For this review, take the finished solid that the model builds, in its own axes (mm). A direction names the side the tool comes from. Give positions to 0.01 mm unless a question says otherwise; leave off trailing zeros. Order: outer loops, then holes, each group sorted by start corner. A loop starts at its lowest first (then second) coordinate and runs counter-clockwise, first axis right, second up. Notation, with made-up numbers: (81.5, -5) -> (130.5, -5) arc R16 ccw to (130.5, 22) -> close; hole circle Ø3 at (46.25, 34.25). An arc over 180 degrees is marked (long way). Return JSON: item names as keys, results as strings. Group by question number.
1) Add section A-A (x = 58.5). Give the boundary of the cut face in (y, z).
2) Insertion check: P1, Ø10, axis at x = 25, y = 1.5, coming from the -Z side; P2, Ø2.5, axis at x = 59.5, z = -1, coming from the +Y side; P3, Ø1.5, axis at x = 40, z = -7, coming from the -Y side; P4, Ø4, axis at x = 51.5, z = 7.5, coming from the +Y side. Each pin has a flat end and moves straight along its axis. Give the tip position at first contact, or say it passes through.
3) Add section B-B (x = 29.5). Give the boundary of the cut face in (y, z) (1 decimal).
4) To check wall thickness, follow line 1 along X through (y, z) = (5, 3.25); line 2 along Y through (x, z) = (40, 0); line 3 along X through (y, z) = (-7.5, -1.5). State the ranges of each line that lie inside material, in increasing order.
5) The part is to be moulded in two halves that separate along Z. For faces 1 (the face through (55.959, 0, 5)), 2 (the face through (39.7, 6.92, -2.41)), 3 (the face through (55.76, 4.65, -1.03)), say which applies: released by +Z, released by -Z, zero draft, split by the parting line, or undercut.
6) For faces 4 (the face through (58.307, 3.219, -5.474)), 5 (the face through (58.307, -3.131, -5.525)), 6 (the face through (5.398, 0, 0)), 7 (the face through (53.578, -2, 10)), 8 (the face through (0, 4, 4)), list the 3-axis set-ups (+Z, -Z, +X, -X, +Y, -Y) from which the entire face can be reached by the end or side of a thin tool; tool diameter is ignored.
from build123d import *

# Parameters (mm, degrees)
CUT_EXTRUDE1_START = -5.0165
SKETCH2_R          = 8.745419401
CUT_EXTRUDE1_DEPTH = 5.0165
SKETCH3_R          = 2.413
CUT_EXTRUDE2_DEPTH = 11.557
SKETCH4_R          = 3.556
CUT_EXTRUDE3_DEPTH = 62.865


with BuildPart() as part:
    # Sketch1 → Revolve1 (revolve)
    with BuildSketch(Plane.XY, mode=Mode.PRIVATE) as revolve1_sk:
        Polygon((2.24506403, 11.1125), (0, 8.86743597), (0, 4.7625), (-3.175, 4.7625), (-3.175, 0), (0, 0), (55.5625, 0), (68.2625, 0), (68.2625, 5.1435), (60.721875, 5.1435), (60.721875, 8.745419401), (55.959375, 8.745419401), (55.959375, 4.7625), (55.5625, 4.7625), (55.5625, 11.1125), (53.975, 11.1125), (53.975, 10.004904014), (53.578125, 10.004904014), (53.578125, 11.1125), align=None)
    revolve(revolve1_sk.sketch.rotate(Axis((0, 0, 0), (1, 0, 0)), 90), axis=Axis((0, 0, 0), (1, 0, 0)))

    # Sketch2 → Cut-Extrude1 (cut)
    with BuildSketch(Plane(origin=(60.721875, 0, 0), x_dir=(0, 0, -1), z_dir=(1, 0, 0)).offset(CUT_EXTRUDE1_START)):
        Circle(SKETCH2_R)
        Polygon((-3.666174209, 6.35), (3.666174209, 6.35), (7.332348419, 0), (3.666174209, -6.35), (-3.666174209, -6.35), (-7.332348419, 0), align=None, mode=Mode.SUBTRACT)
    extrude(amount=CUT_EXTRUDE1_DEPTH, mode=Mode.SUBTRACT)

    # Sketch3 → Cut-Extrude2 (cut)
    with BuildSketch(Plane(origin=(0, 11.1125, 0), x_dir=(1, 0, 0), z_dir=(0, 1, 0))):
        with Locations(Location((39.590311937, 0, 0), (0, 0, 270))):
            Circle(SKETCH3_R)
    extrude(amount=-CUT_EXTRUDE2_DEPTH, mode=Mode.SUBTRACT)

    # Sketch4 → Cut-Extrude3 (cut)
    with BuildSketch(Plane(origin=(68.2625, 0, 0), x_dir=(0, 0, -1), z_dir=(1, 0, 0))):
        Circle(SKETCH4_R)
    extrude(amount=-CUT_EXTRUDE3_DEPTH, mode=Mode.SUBTRACT)


solid = part.part
Evaluation:
{
 "1": {"outline": "(-6.35, -3.67) -> (0, -7.33) -> (6.35, -3.67) -> (6.35, 3.67) -> (0, 7.33) -> (-6.35, 3.67) -> close; hole circle Ø7.11 at (0, 0)"},
 "2": {"P1": "z = -11.11", "P2": "y = 6.35", "P3": "y = -9.19", "P4": "y = 9.66"},
 "3": {"outline": "circle Ø22.2 at (0, 0); hole circle Ø7.1 at (0, 0)"},
 "4": {"line 1": "0 to 55.56, 55.96 to 60.72", "line 2": "-11.11 to -3.56", "line 3": "0 to 55.56"},
 "5": {"face 1": "zero draft", "face 2": "undercut", "face 3": "split by the parting line"},
 "6": {"face 4": "-Z, +X, +Y", "face 5": "-Z, +X, -Y", "face 6": "+X", "face 7": "none", "face 8": "-X"}
}
